from build123d import *

# Parameters (mm, degrees)
BLANKSKE_W          = 120
BLANKSKE_H          = 16
BLANK_DEPTH         = 8
TOOTHCUTSIM_DEPTH   = 122.326007105
TEETHCUTS_COUNT     = 20
TEETHCUTS_PITCH     = 6.2831853
SKETCH1_W           = 8
SKETCH1_H           = 1
CUT_EXTRUDE1_DEPTH  = 122.326007105
BOSS_EXTRUDE2_DEPTH = 8
CUT_EXTRUDE2_DEPTH  = 170.803562978


with BuildPart() as part:
    # BlankSke → Blank (new body)
    with BuildSketch(Plane.XY):
        with Locations((60, 8)):
            Rectangle(BLANKSKE_W, BLANKSKE_H)
    extrude(amount=-BLANK_DEPTH)

    # TooCutSkeSim → ToothCutSim (cut, through all)
    with BuildSketch(Plane.XY):
        Polygon((0.861870739, 11.5), (-0.861870739, 11.5), (-2.508981637, 16.0254), (2.508981637, 16.0254), align=None)
    toothcutsim = extrude(amount=-TOOTHCUTSIM_DEPTH, mode=Mode.SUBTRACT)

    # TeethCuts: ToothCutSim ×20
    with Locations(*[(i * TEETHCUTS_PITCH, 0, 0) for i in range(1, TEETHCUTS_COUNT)]):
        add(toothcutsim, mode=Mode.SUBTRACT)

    # Sketch1 → Cut-Extrude1 (cut, through all)
    with BuildSketch(Plane(origin=(120, 0, 0), x_dir=(0, 0, -1), z_dir=(1, 0, 0))):
        with Locations((4, 0.5)):
            Rectangle(SKETCH1_W, SKETCH1_H)
    extrude(amount=-CUT_EXTRUDE1_DEPTH, mode=Mode.SUBTRACT)

    # Sketch3 → Boss-Extrude2 (add)
    with BuildSketch(Plane.ZY):
        Polygon((0, 1), (15.5, 1), (15.5, -39), (95.5, -39), (95.5, -9), (35.5, 61), (15.5, 61), (15.5, 10.5), (0, 10.5), align=None)
    extrude(amount=-BOSS_EXTRUDE2_DEPTH)

    # Sketch4 → Cut-Extrude2 (cut, through all)
    with BuildSketch(Plane(origin=(0, 0, -8), x_dir=(-1, 0, 0), z_dir=(0, 0, -1))):
        Polygon((-120, 11.5), (-118.518649961, 11.5), (-116.880783906, 16), (-115.597072194, 16), (-113.959206139, 11.5), (-113.218706139, 11.5), (-112.235464661, 11.5), (-110.597598606, 16), (-109.313886894, 16), (-107.676020839, 11.5), (-105.952279361, 11.5), (-104.314413306, 16), (-103.030701594, 16), (-101.392835539, 11.5), (-99.669094061, 11.5), (-98.031228006, 16), (-96.747516294, 16), (-95.109650239, 11.5), (-93.385908761, 11.5), (-91.748042706, 16), (-90.464330994, 16), (-88.826464939, 11.5), (-87.102723461, 11.5), (-85.464857406, 16), (-84.181145694, 16), (-82.543279639, 11.5), (-80.819538161, 11.5), (-79.181672106, 16), (-77.897960394, 16), (-76.260094339, 11.5), (-75.3982236, 11.5), (-75.3982236, 1), (-76.260094339, 1), (-101.392835539, 1), (-113.218706139, 1), (-120, 1), align=None)
    extrude(amount=-CUT_EXTRUDE2_DEPTH, mode=Mode.SUBTRACT)


solid = part.part
Model file for the job. Use its own axes, mm. A direction names the side the tool comes from. Coordinates: 2 decimals unless noted, no trailing zeros. Order: outer loops, then holes, each group sorted by start corner. A loop starts at its lowest first (then second) coordinate and runs counter-clockwise, first axis right, second up. Notation, with made-up numbers: (-17.5, 10.25) -> (25.5, 10.25) arc R27 ccw to (25.5, 38.25) -> close; hole circle Ø8 at (33.5, 58). An arc over 180 degrees is marked (long way). Return JSON: item names as keys, results as strings. Group by question number.
Item 1: Flat gauge pins, fed straight in: P1, Ø4.5, axis at x = 45.5, y = 8, coming from the +Z side; P2, Ø2.5, axis at x = 4.5, y = -20, coming from the -Z side; P3, Ø0.6, axis at x = 41, z = -3, coming from the +Y side. Where does each tip first touch, or does it go through?
Item 2: Pull direction X, two halves, no side cores. Call faces 1 (the flat face through (0, 1, 43)), 2 (the flat face through (8, 1, 47)), 3 (the flat face through (36.03, 13.72, -3.94)), 4 (the flat face through (3.94, 25.51, 65.92)): pulls with the +X half, pulls with the -X half, needs draft (parallel to the pull), parting line crosses it, or undercut.
Item 3: Saw through at A-A on z = 24. Write the cut outline in (x, y), then the cut area to 3 significant figures.
Item 4: Saw through at C-C on z = 50.5. Write the cut outline in (x, y).
Item 5: Saw through at B-B on y = 8. Write the cut outline in (x, z), then the cut area to 3 significant figures.
Item 6: Wall check: line 1 along X through (y, z) = (15, 59); line 2 along Y through (x, z) = (41, -0.5); line 3 along Z through (x, y) = (32.5, 11.5). Give the ranges that are in metal, low to high. Write a range as [from, to].
Item 7: Tool access for faces 5 (the flat face through (1.7, 13.8, -3.9)), 6 (the flat face through (29, 1, -2)), 7 (the flat face through (64.524, 13.782, -3.944)): list every direction of +Z, -Z, +X, -X, +Y, -Y with a clear straight run to the whole face (end or side of a thin tool).
Values found:
{
 "1": {"P1": "stops at z = 0", "P2": "stops at z = 15.5", "P3": "stops at y = 16"},
 "2": {"face 1": "pulls with the -X half", "face 2": "pulls with the +X half", "face 3": "undercut", "face 4": "needs draft"},
 "3": {"outline": "(0, -39) -> (8, -39) -> (8, 61) -> (0, 61) -> close", "area": "800 mm2"},
 "4": {"outline": "(0, -39) -> (8, -39) -> (8, 43.5) -> (0, 43.5) -> close"},
 "5": {"outline": "(0, -8) -> (75.4, -8) -> (75.4, 0) -> (8, 0) -> (8, 80.93) -> (0, 80.93) -> close", "area": "1,250 mm2"},
 "6": {"line 1": "x = [0, 8]", "line 2": "y = [1, 16]", "line 3": "z = [-8, 0]"},
 "7": {"face 5": "-Z, -X, +Y", "face 6": "-Z, +X, -X, -Y", "face 7": "+Z, -Z, +Y"}
}
